For this review, take the finished solid that the model builds, in its own axes (mm). A direction names the side the tool comes from. Coordinates: 2 decimals unless noted, no trailing zeros. Write each loop counter-clockwise with the first axis right and the second up, starting at its lowest first coordinate (ties: lowest second). Pieces come first, ordered by that corner, then holes.
1) Mouldability with a two-part tool opening along X and no side actions: class faces 1 (the face through (-39.365, 61.689, -0.133)), 2 (the face through (60.325, 0, 40)) as pulls with the +X half, pulls with the -X half, needs draft (parallel to the pull), parting line crosses it, or undercut.
2) To check wall thickness, follow line 1 along X through (y, z) = (15, 20) (3 decimals); line 2 along Z through (x, y) = (21.5, 33) (3 decimals); line 3 along Y through (x, z) = (-14.5, 37.5). State the ranges of each line that lie inside material, in increasing order.
3) Insertion check: P1, Ø5, axis at y = 16, z = 20.5, coming from the -X side (3 decimals); P2, Ø17, axis at x = 58, z = 24.5, coming from the -Y side; P3, Ø15, axis at x = 86, y = -10.5, coming from the -Z side; P4, Ø12, axis at y = -1.5, z = 30, coming from the -X side. Each pin has a flat end and moves straight along its axis. Give the tip position at first contact, or say it passes through.
4) We need section A-A on z = -0.5. Write out the cut boundary in (x, y) (3 decimals), then the cut area to 3 significant figures.
5) We need section B-B on x = 81.5. Write out the cut boundary in (y, z) (3 decimals).
6) For faces 3 (the face through (54, 25.4, 45)), 4 (the face through (86, 0, 38.1)), 5 (the face through (60.325, 0, 64)), list the 3-axis set-ups (+Z, -Z, +X, -X, +Y, -Y) from which the entire face can be reached by the end or side of a thin tool; tool diameter is ignored.
7) We need section C-C on y = 31. Write out the cut boundary in (x, z) (3 decimals), then the cut area to 3 significant figures.
from build123d import *

# Parameters (mm, degrees)
F1_DEPTH = 63.5
F0_W     = 25.4
F0_H     = 4.7752
F0_H_2   = 4.7256098347
F0_H_3   = 19.0741901653
F2_DEPTH = 25.4
F3_DEPTH = 7.9375
F5_R     = 6.35


with BuildPart() as f1:
    # F0 (on Front) → F1 (new body, symmetric)
    with BuildSketch(Plane.XZ):
        Polygon((-41.275, 9.525), (-41.275, -9.525), (41.275, -9.525), (41.275, 9.525), (22.225, 9.525), align=None)
    extrude(amount=F1_DEPTH, both=True)

    # F0 (on Front) → F2 (join, symmetric)
    with BuildSketch(Plane.XZ):
        Polygon((-41.275, 9.525), (-41.275, -9.525), (41.275, -9.525), (41.275, 9.525), (22.225, 9.525), align=None)
        with Locations((73.025, 40.4876)):
            Rectangle(F0_W, F0_H)
        with Locations((73.025, 64.3121950827)):
            Rectangle(F0_W, F0_H_2)
        with BuildLine():
            Line((22.225, 9.525), (41.275, 9.525))
            Line((41.275, 9.525), (41.275, 27.1020599752))
            ThreePointArc((41.275, 27.1020599752), (46.5785126871, 38.9451710949), (58.9454605977, 42.8752))
            Line((58.9454605977, 42.8752), (60.325, 42.8752))
            Line((60.325, 42.8752), (60.325, 61.9493901653))
            Line((60.325, 61.9493901653), (54.8220816984, 61.9493901653))
            ThreePointArc((54.8220816984, 61.9493901653), (31.6445283156, 50.9605288942), (22.225, 27.1020599752))
            Line((22.225, 27.1020599752), (22.225, 9.525))
        make_face()
        with Locations((73.025, 52.4122950827)):
            Rectangle(F0_W, F0_H_3)
    extrude(amount=F2_DEPTH, both=True)

    # F0 (on Front) → F3 (join, symmetric)
    with BuildSketch(Plane.XZ):
        with BuildLine():
            add(Edge.make_bspline(
                [(-41.275, 9.525), (-22.719591856, 45.2046655118), (17.2888338566, 62.9861876369), (54.8220816984, 61.9493901653)],
                knots=[0, 0, 0, 0, 109.4667337375, 109.4667337375, 109.4667337375, 109.4667337375], degree=3))
            Line((-41.275, 9.525), (22.225, 9.525))
            Line((22.225, 9.525), (22.225, 27.1020599752))
            ThreePointArc((22.225, 27.1020599752), (31.6445283156, 50.9605288942), (54.8220816984, 61.9493901653))
        make_face()
    extrude(amount=F3_DEPTH, both=True)

    # F0 (on Front) → F4 (revolve)
    with BuildSketch(Plane.XZ):
        Polygon((85.725, 66.675), (85.725, 61.9493901653), (85.725, 42.8752), (85.725, 38.1), (111.125, 38.1), (111.125, 66.675), align=None)
    revolve(axis=Axis((85.725, 0, 52.3875), (0, 0, -1)))

    # F5
    f5_edges = [f1.edges().sort_by_distance(p)[0] for p in [
        (41.275, -63.5, 0),
        (-41.275, -63.5, 0),
        (-41.275, 63.5, 0),
        (41.275, 63.5, 0),
    ]]
    fillet(f5_edges, radius=F5_R)


solid = f1.part
Result:
1. face 1: pulls with the -X half
1. face 2: undercut
2. line 1: x = 22.225 to 41.275
2. line 2: z = -9.525 to 9.525
2. line 3: y = -7.94 to 7.94
3. P1: stops at x = 22.225
3. P2: passes through
3. P3: stops at z = 38.1
3. P4: stops at x = -31.85
4. outline: (-41.275, -57.15) arc R6.35 ccw to (-34.925, -63.5) - (34.925, -63.5) arc R6.35 ccw to (41.275, -57.15) - (41.275, 57.15) arc R6.35 ccw to (34.925, 63.5) - (-34.925, 63.5) arc R6.35 ccw to (-41.275, 57.15) - close
4. area: 10,400 mm2
5. outline: (-25.4, 38.1) - (25.4, 38.1) - (25.4, 66.675) - (-25.4, 66.675) - close
6. face 3: +Z, +X, -X, +Y
6. face 4: -Z, +X, +Y, -Y
6. face 5: +Z, -X, +Y, -Y
7. outline: (-41.275, -9.525) - (41.275, -9.525) - (41.275, 9.525) - (-41.275, 9.525) - close
7. area: 1,570 mm2
